```python
from build123d import *

# Parameters (mm, degrees)
F0_R     = 1.5875
F1_DEPTH = 304.8


# Not quite as in the source:
# - ends of sketch curves that miss each other by under 0.0002 mm in the source are joined


with BuildPart() as f1:
    # F0 (on Front) → F1 (new body)
    with BuildSketch(Plane.XZ):
        with BuildLine():
            Line((0, -35.9251248209), (0, -42.2751248896))
            ThreePointArc((0, -42.2751248896), (2.2450640303, -43.2050608593), (3.175, -45.4501248896))
            Line((3.175, -45.4501248896), (9.5250000687, -45.4501248896))
            ThreePointArc((9.5250000687, -45.4501248896), (6.7351921394, -38.7149327502), (0, -35.9251248209))
        make_face()
        with BuildLine():
            ThreePointArc((3.175, -45.4501248896), (-2.2450640303, -47.6951889199), (0, -42.2751248896))
            Line((0, -42.2751248896), (0, -35.9251248209))
            ThreePointArc((0, -35.9251248209), (-6.6836697304, -38.6638014929), (-9.5238937406, -45.3049548981))
            ThreePointArc((-9.5238937406, -45.3049548981), (-6.7863233967, -52.13379462), (0, -54.9751249583))
            Line((0, -54.9751249583), (0.6773435819, -54.951010742))
            ThreePointArc((0.6773435819, -54.951010742), (6.9705567917, -51.941424014), (9.5250000687, -45.4501248896))
            Line((9.5250000687, -45.4501248896), (3.175, -45.4501248896))
        make_face()
        with BuildLine():
            Line((36.5125, -45.4501248896), (9.5250000687, -45.4501248896))
            ThreePointArc((9.5250000687, -45.4501248896), (6.9705567917, -51.941424014), (0.6773435819, -54.951010742))
            Line((0.6773435819, -54.951010742), (44.7324052867, -53.3825995038))
            ThreePointArc((44.7324052867, -53.3825995038), (38.9380895197, -51.1617576778), (36.5125, -45.4501248896))
        make_face()
        with BuildLine():
            Line((0, -4.1751248896), (0, -35.9251248209))
            ThreePointArc((0, -35.9251248209), (6.7351921394, -38.7149327502), (9.5250000687, -45.4501248896))
            Line((9.5250000687, -45.4501248896), (36.5125, -45.4501248896))
            ThreePointArc((36.5125, -45.4501248896), (38.9380895197, -39.7384921015), (44.7324052867, -37.5176502755))
            Line((44.7324052867, -37.5176502755), (19.1378694473, -36.6064551461))
            ThreePointArc((19.1378694473, -36.6064551461), (13.3988872221, -33.8519658653), (11.5206935861, -27.7695718592))
            Line((11.5206935861, -27.7695718592), (15.7748262706, 9.9192906189))
            ThreePointArc((15.7748262706, 9.9192906189), (10.5770706294, -0.1382498214), (0, -4.1751248896))
        make_face()
        with BuildLine():
            ThreePointArc((-9.5238937406, -45.3049548981), (-6.6836697304, -38.6638014929), (0, -35.9251248209))
            Line((0, -35.9251248209), (0, -4.1751248896))
            ThreePointArc((0, -4.1751248896), (-10.5752191937, -0.1399037729), (-15.7742685853, 9.9143568106))
            Line((-15.7742685853, 9.9143568106), (-9.5238937406, -45.3049548981))
        make_face()
        with BuildLine():
            ThreePointArc((-15.7038062969, 14.0249757078), (-10.370743778, 23.7191637121), (0, 27.5748751104))
            Line((0, 27.5748751104), (0, 47.8104427457))
            Line((0, 47.8104427457), (0, 59.3248751104))
            ThreePointArc((0, 59.3248751104), (-7.0846213328, 62.4832617586), (-9.4708755422, 69.8638482188))
            Line((-9.4708755422, 69.8638482188), (-15.7038062969, 14.0249757078))
        make_face()
        with Locations((-2.6159647387, 47.8104427457)):
            Circle(F0_R, mode=Mode.SUBTRACT)
        with BuildLine():
            Line((0, 47.8104427457), (0, 27.5748751104))
            ThreePointArc((0, 27.5748751104), (10.5770706294, 23.5380000422), (15.7748262706, 13.4804596019))
            Line((15.7748262706, 13.4804596019), (9.4660212705, 69.9082069616))
            ThreePointArc((9.4660212705, 69.9082069616), (9.5102438875, 69.3798620908), (9.525, 68.8498751104))
            ThreePointArc((9.525, 68.8498751104), (6.7351920908, 62.1146830196), (0, 59.3248751104))
            Line((0, 59.3248751104), (0, 47.8104427457))
        make_face()
        with BuildLine():
            ThreePointArc((9.4660212705, 69.9082069616), (-0.0223117795, 78.3748489783), (-9.4708755422, 69.8638482188))
            ThreePointArc((-9.4708755422, 69.8638482188), (-7.0846213328, 62.4832617586), (0, 59.3248751104))
            ThreePointArc((0, 59.3248751104), (6.7351920908, 62.1146830196), (9.525, 68.8498751104))
            ThreePointArc((9.525, 68.8498751104), (9.5102438875, 69.3798620908), (9.4660212705, 69.9082069616))
        make_face()
        with BuildLine():
            ThreePointArc((3.175, 68.8498751104), (2.2450640303, 66.6048110801), (0, 65.6748751104))
            ThreePointArc((0, 65.6748751104), (-2.2450640303, 71.0949391407), (3.175, 68.8498751104))
        make_face(mode=Mode.SUBTRACT)
        with BuildLine():
            ThreePointArc((44.7324052867, -37.5176502755), (38.9380895197, -39.7384921015), (36.5125, -45.4501248896))
            ThreePointArc((36.5125, -45.4501248896), (38.9380895197, -51.1617576778), (44.7324052867, -53.3825995038))
            ThreePointArc((44.7324052867, -53.3825995038), (50.1616327882, -50.96203537), (52.3875, -45.4501248896))
            ThreePointArc((52.3875, -45.4501248896), (50.1616327882, -39.9382144093), (44.7324052867, -37.5176502755))
        make_face()
        with BuildLine():
            ThreePointArc((47.625, -45.4501248896), (44.45, -48.6251248896), (41.275, -45.4501248896))
            ThreePointArc((41.275, -45.4501248896), (44.45, -42.2751248896), (47.625, -45.4501248896))
        make_face(mode=Mode.SUBTRACT)
        with BuildLine():
            Line((0, 8.5248751104), (0, -4.1751248896))
            ThreePointArc((0, -4.1751248896), (10.5770706294, -0.1382498214), (15.7748262706, 9.9192906189))
            ThreePointArc((15.7748262706, 9.9192906189), (15.8499367829, 10.8081750617), (15.875, 11.6998751104))
            ThreePointArc((15.875, 11.6998751104), (15.8499367829, 12.5915751591), (15.7748262706, 13.4804596019))
            ThreePointArc((15.7748262706, 13.4804596019), (10.5770706294, 23.5380000422), (0, 27.5748751104))
            Line((0, 27.5748751104), (0, 14.8748751104))
            ThreePointArc((0, 14.8748751104), (2.2450640303, 13.9449391407), (3.175, 11.6998751104))
            ThreePointArc((3.175, 11.6998751104), (2.2450640303, 9.4548110801), (0, 8.5248751104))
        make_face()
        with BuildLine():
            ThreePointArc((-15.7742685853, 9.9143568106), (-10.5752191937, -0.1399037729), (0, -4.1751248896))
            Line((0, -4.1751248896), (0, 8.5248751104))
            ThreePointArc((0, 8.5248751104), (-3.175, 11.6998751104), (0, 14.8748751104))
            Line((0, 14.8748751104), (0, 27.5748751104))
            ThreePointArc((0, 27.5748751104), (-10.370743778, 23.7191637121), (-15.7038062969, 14.0249757078))
            Line((-15.7038062969, 14.0249757078), (-15.8299773584, 12.8946310826))
            ThreePointArc((-15.8299773584, 12.8946310826), (-15.8722272886, 11.4031835217), (-15.7742685853, 9.9143568106))
        make_face()
    extrude(amount=F1_DEPTH)


solid = f1.part
```
Model file for the job. Use its own axes, mm. A direction names the side the tool comes from. Give positions to 0.01 mm unless a question says otherwise; leave off trailing zeros. Loops run counter-clockwise (first coordinate to the right, second up) from the corner with the lowest first, then second, coordinate; pieces in that order, holes last. Notation, with made-up numbers: (26, 77) - (83, 77) arc R17 ccw to (83, 95) - close; hole circle Ø9 at (-34.5, -31.5). An arc over 180 degrees is marked (long way). One line per item, written item: value. Start each with the question number.
1. Slice it at C-C (z = 1). List the corners of the cut face in (x, y).
2. Probe L1, parallel to Z at x = 0.5, y = -267.5; L2, parallel to Z at x = 2, y = -138; L3, parallel to Z at x = 47, y = -92. List the from-to ranges inside material, lowest first. Write a range as from..to.
3. Slice it at B-B (x = 28.5). List the corners of the cut face in (y, z).
4. Pin check, flat tips, straight feed: pin 1 (5.5 mm diameter, centred on x = 0, z = -45.45, fed in from +Y); pin 2 (1 mm diameter, centred on x = 33.5, z = -37, fed in from +Y); pin 3 (1.5 mm diameter, centred on x = 9, y = -184, fed in from +Z); pin 4 (2 mm diameter, centred on x = 20.5, y = -268, fed in from -Z). Stop position of each tip, or through.
5. Pull direction Z, two halves, no side cores. Call faces 3 (the flat face through (13.618, -150.266, -9.189)), 4 (the flat face through (12.665, -150.266, 41.299)), 5 (the flat face through (-12.693, -150.266, -17.309)): pulls with the +Z half, pulls with the -Z half, needs draft (parallel to the pull), parting line crosses it, or undercut.
6. Slice it at A-A (y = -142). Give the number of separate pieces and of enclosed holes in the cut face, plus the area to 3 significant figures.
7. Which spindle directions (+Z, -Z, +X, -X, +Y, -Y) get a long thin tool onto all of the face, cutting with end or side? Do faces 1 (the cylindrical face through (41.52, -150.27, -46.67)), 2 (the cylindrical face through (13.46, -150.27, -33.92)). Say none if no direction does.
Solution:
1. outline: (-14.77, -304.8) - (14.77, -304.8) - (14.77, 0) - (-14.77, 0) - close
2. L1: z = -54.96..-48.59, -42.31..8.56, 14.84..65.71, 71.99..78.36
2. L2: z = -54.9..-47.92, -42.98..9.23, 14.17..66.38, 71.32..78.16
2. L3: z = -52.97..-47.34, -43.56..-37.93
3. outline: (-304.8, -53.96) - (0, -53.96) - (0, -36.94) - (-304.8, -36.94) - close
4. pin 1: passes through
4. pin 2: stops at y = 0
4. pin 3: stops at z = 73.61
4. pin 4: stops at z = -54.28
5. face 3: undercut
5. face 4: pulls with the +Z half
5. face 5: pulls with the -Z half
6. separate pieces: 1
6. enclosed holes: 5
6. area: 3,790 mm^2
7. face 1: +Y, -Y
7. face 2: +X, +Y, -Y
